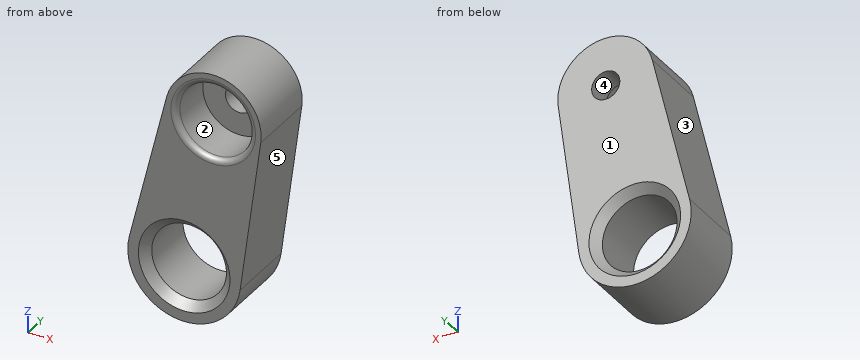
```python
from build123d import *

# Parameters (mm, degrees)
SKETCH1_R           = 2.6
SKETCH1_R_2         = 2.65
BOSS_EXTRUDE1_DEPTH = 3.2
BOSS_EXTRUDE2_START = 3.2
SKETCH1_3_R         = 2.65
SKETCH1_3_R_2       = 1
BOSS_EXTRUDE2_DEPTH = 1.8
CHAMFER1_SIZE       = 0.6
FILLET3_R           = 0.4


with BuildPart() as part:
    # Sketch1 → Boss-Extrude1 (new body)
    with BuildSketch(Plane(origin=(0, 33, 0), x_dir=(1, 0, 0), z_dir=(0, 1, 0))):
        with BuildLine():
            Line((5.429968705, -10.516152569), (3.965267434, 0.525979253))
            ThreePointArc((3.965267434, 0.525979253), (-0.738499825, 3.931236194), (-3.885823258, -0.948882295))
            Line((-3.885823258, -0.948882295), (-1.243458383, -11.769784885))
            ThreePointArc((-1.243458383, -11.769784885), (2.687216237, -14.304785699), (5.429968705, -10.516152569))
        make_face()
        with Locations(Location((2.059491386, -10.963234935, 0), (0, 0, 270))):
            Circle(SKETCH1_R, mode=Mode.SUBTRACT)
        with Locations(Location((0, 0, 0), (0, 0, 270))):
            Circle(SKETCH1_R_2, mode=Mode.SUBTRACT)
    extrude(amount=BOSS_EXTRUDE1_DEPTH)

    # Sketch1<3> → Boss-Extrude2 (add)
    with BuildSketch(Plane(origin=(0, 33, 0), x_dir=(1, 0, 0), z_dir=(0, 1, 0)).offset(BOSS_EXTRUDE2_START)):
        with BuildLine():
            Line((5.429968705, -10.516152569), (3.965267434, 0.525979253))
            ThreePointArc((3.965267434, 0.525979253), (-0.738499825, 3.931236194), (-3.885823258, -0.948882295))
            Line((-3.885823258, -0.948882295), (-1.243458383, -11.769784885))
            ThreePointArc((-1.243458383, -11.769784885), (2.687216237, -14.304785699), (5.429968705, -10.516152569))
        make_face()
        with Locations(Location((0, 0, 0), (0, 0, 270))):
            Circle(SKETCH1_3_R, mode=Mode.SUBTRACT)
        with Locations(Location((2.059491386, -10.963234935, 0), (0, 0, 270))):
            Circle(SKETCH1_3_R_2, mode=Mode.SUBTRACT)
    extrude(amount=BOSS_EXTRUDE2_DEPTH)

    # Chamfer1
    chamfer1_edges = [part.edges().sort_by_distance(p)[0] for p in [
        (0, 33, -2.65),
        (0, 38, -2.65),
    ]]
    chamfer(chamfer1_edges, length=CHAMFER1_SIZE)

    # Fillet3
    fillet3_edges = [part.edges().sort_by_distance(p)[0] for p in [
        (2.059491386, 33, 8.363234935),
    ]]
    fillet(fillet3_edges, radius=FILLET3_R)


solid = part.part
```
For this review, take the finished solid that the model builds, in its own axes (mm). Face numbers are marked on the shaded views. A direction names the side the tool comes from. Coordinates: 2 decimals unless noted, no trailing zeros. Order: outer loops, then holes, each group sorted by start corner. A loop starts at its lowest first (then second) coordinate and runs counter-clockwise, first axis right, second up. Notation, with made-up numbers: (45.5, 57) -> (76.5, 57) arc R18 cw to (76.5, 83) -> close; hole circle Ø5 at (62.25, 18). An arc over 180 degrees is marked (long way). Answer as CSV lines item,"result".
Q1. We need section C-C (x = 1.75). Count the separate pieces of the cut face and the enclosed holes in it, plus the area to 3 significant figures.
Model answer:
separate pieces,"3"
enclosed holes,"0"
area,"48.9 mm2"
Q2. For the marked faces 1 and 2, list the 3-axis set-ups (+Z, -Z, +X, -X, +Y, -Y) from which the entire face can be reached by the end or side of a thin tool; tool diameter is ignored.
Model answer:
face 1,"+Z, -Z, +X, -X, +Y"
face 2,"-Y"
Q3. Wall thickness on line 1 along Z through (x, y) = (2.25, 34.65); line 2 along Z through (x, y) = (1.25, 35.7); line 3 along X through (y, z) = (36, 11.25): over which ranges is each line inside the solid? List them lowest first. Write a range as [from, to].
Model answer:
line 1,"z = [-3.31, -1.4], [1.4, 8.37], [13.56, 14.36]"
line 2,"z = [-3.8, -2.34], [2.34, 8.49], [13.43, 14.27]"
line 3,"x = [-1.37, -0.52], [4.64, 5.45]"
Q4. Draft analysis for pull direction X (two halves, no side actions). For the marked faces 3, 4 and 5, state which applies: released by +X, released by -X, zero draft, split by the parting line, or undercut.
Model answer:
face 3,"released by -X"
face 4,"undercut"
face 5,"released by +X"
Q5. We need section A-A (z = 0). State the section outline as (x, y) points.
Model answer:
outline,"(-4, 33) -> (-3.25, 33) -> (-2.65, 33.6) -> (-2.65, 37.4) -> (-3.25, 38) -> (-4, 38) -> close; (2.65, 33.6) -> (3.25, 33) -> (4.04, 33) -> (4.04, 38) -> (3.25, 38) -> (2.65, 37.4) -> close"
Q6. Clearance check with flat-ended pins moving along their axes: pin 1 Ø3 at (x, y) = (0, 34) entering from +Z; pin 2 Ø4.5 at (x, z) = (2.06, 10.96) entering from -Y. State where each tip first meets the part, or that it passes through.
Model answer:
pin 1,"stops at z = 14.32"
pin 2,"stops at y = 36.2"
